from build123d import *

# Parameters (mm, degrees)
ESQUISSE1_W             = 150
ESQUISSE1_H             = 100
BOSS_EXTRU_1_DEPTH      = 3
CONG_1_R                = 1
D_GAGEMENT_M31_D        = 3.4
D_GAGEMENT_M31_DEPTH    = 5
D_GAGEMENT_M31_TIP      = 1.021463052
ESQUISSE4_W             = 10
ESQUISSE4_H             = 3
ENL_V_MAT_EXTRU_1_DEPTH = 3


with BuildPart() as part:
    # Esquisse1 → Boss.-Extru.1 (new body)
    with BuildSketch(Plane(origin=(0, 0, 0), x_dir=(1, 0, 0), z_dir=(0, 1, 0))):
        Rectangle(ESQUISSE1_W, ESQUISSE1_H)
    extrude(amount=BOSS_EXTRU_1_DEPTH)

    # Congé1
    cong_1_edges = [part.edges().sort_by_distance(p)[0] for p in [
        (-75, 3, 0),
        (0, 3, 50),
        (75, 3, 0),
        (0, 0, 50),
        (-75, 0, 0),
        (0, 0, -50),
        (75, 0, 0),
        (0, 3, -50),
        (75, 1.5, 50),
        (-75, 1.5, 50),
        (-75, 1.5, -50),
        (75, 1.5, -50),
    ]]
    fillet(cong_1_edges, radius=CONG_1_R)

    # Dégagement M31
    with Locations(Plane(origin=(0, 3, 0), x_dir=(-1, 0, 0), z_dir=(0, 1, 0))):
        with Locations((67.5, 42.113248654), (-67.5, 42.113248654), (-67.5, -42.113248654), (67.5, -42.113248654)):
            Hole(D_GAGEMENT_M31_D / 2, depth=D_GAGEMENT_M31_DEPTH)
            with Locations((0, 0, -(D_GAGEMENT_M31_DEPTH + D_GAGEMENT_M31_TIP / 2))):  # 118° drill point
                Cone(0, D_GAGEMENT_M31_D / 2, D_GAGEMENT_M31_TIP, mode=Mode.SUBTRACT)

    # Esquisse4 → Enlèv. mat.-Extru.1 (cut)
    with BuildSketch(Plane(origin=(0, 3, 0), x_dir=(1, 0, 0), z_dir=(0, 1, 0))):
        with Locations((0, 24.5)):
            Rectangle(ESQUISSE4_W, ESQUISSE4_H)
        with Locations((0, -24.5)):
            Rectangle(ESQUISSE4_W, ESQUISSE4_H)
    extrude(amount=-ENL_V_MAT_EXTRU_1_DEPTH, mode=Mode.SUBTRACT)


solid = part.part
For this review, take the finished solid that the model builds, in its own axes (mm). A direction names the side the tool comes from. Coordinates: 2 decimals unless noted, no trailing zeros. Order: outer loops, then holes, each group sorted by start corner. A loop starts at its lowest first (then second) coordinate and runs counter-clockwise, first axis right, second up. Notation, with made-up numbers: (50.25, 26.25) - (73.25, 26.25) arc R22 ccw to (73.25, 55.25) - close; hole circle Ø11 at (55, 63). An arc over 180 degrees is marked (long way). Answer as CSV lines item,"result". Start each with the question number.
1) Add section A-A (x = -67.5). State the section outline as (y, z) points, then the cut area to 3 significant figures.
2) Draft analysis for pull direction Z (two halves, no side actions). For faces 1 (the flat face through (0, 2, -23)), 2 (the flat face through (-1, 3, -1)), state which applies: +Z half, -Z half, draft (parallel to the pull), parting line (faces both ways), or undercut.
3) Insertion check: P1, Ø2.5, axis at x = 67.5, z = 42.11, coming from the +Y side. The pin has a flat end and moves straight along its axis. Give the tip position at first contact, or say it passes through.
4) Machinability: for faces 3 (the flat face through (-1, 0, -1)), 4 (the flat face through (-5, 2, -24)), which of the approach directions +Z, -Z, +X, -X, +Y, -Y give a long, thin tool a straight path to every point of the face, cutting with its end or side? Answer none if there is none.
5) To check wall thickness, follow line 1 along Z through (x, y) = (-67.5, 2.1); line 2 along Z through (x, y) = (1.5, 1.85); line 3 along X through (y, z) = (0.8, 2.5). State the ranges of each line that lie inside material, in increasing order. Write a range as [from, to].
Result:
1,outline,"(0, -49) arc R1 ccw to (1, -50) - (2, -50) arc R1 ccw to (3, -49) - (3, -43.81) - (0, -43.81) - close; (0, -40.41) - (3, -40.41) - (3, 40.41) - (0, 40.41) - close; (0, 43.81) - (3, 43.81) - (3, 49) arc R1 ccw to (2, 50) - (1, 50) arc R1 ccw to (0, 49) - close"
1,area,"279 mm^2"
2,face 1,"undercut"
2,face 2,"draft"
3,P1,"through"
4,face 3,"+Z, -Z, +X, -X, -Y"
4,face 4,"+Y, -Y"
5,line 1,"[-49.99, -43.81], [-40.41, 40.41], [43.81, 49.99]"
5,line 2,"[-50, -26], [-23, 23], [26, 50]"
5,line 3,"[-74.98, 74.98]"
